Can you work these out from the drawing? Everything is in mm from the part's minimum corner. A direction names the side the tool comes from. Round coordinates to 2 decimals unless told otherwise and drop trailing zeros. Loops run counter-clockwise (first coordinate to the right, second up) from the corner with the lowest first, then second, coordinate; pieces in that order, holes last. Notation, with made-up numbers: (14.5, -2) -> (58.5, -2) arc R15 cw to (58.5, 9) -> close; hole circle Ø4 at (39.25, 29). An arc over 180 degrees is marked (long way). One line per item, written item: value.
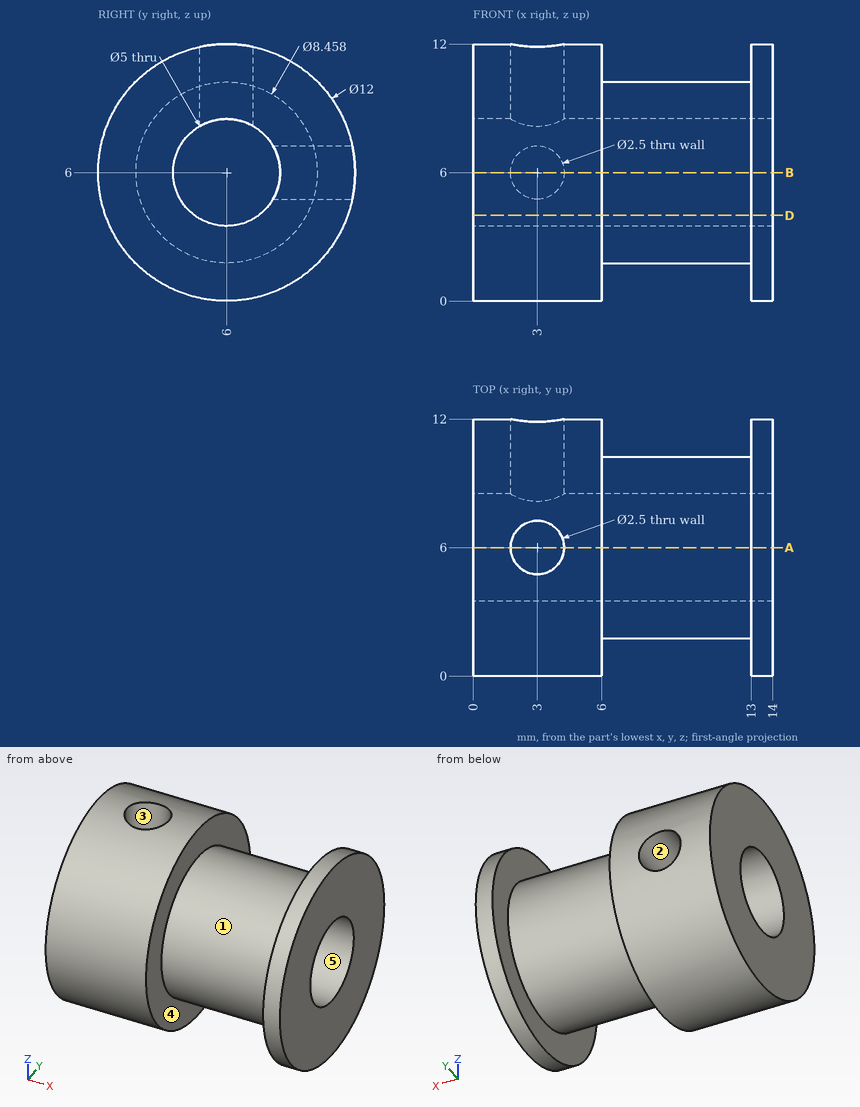
Item 1: If we section it at A-A on y = 6: List the corners of the cut face in (x, z) for me.
Output:
outline: (0, 0) -> (6, 0) -> (6, 1.77) -> (13, 1.77) -> (13, 0) -> (14, 0) -> (14, 3.5) -> (0, 3.5) -> close; (0, 8.5) -> (1.75, 8.5) -> (1.75, 12) -> (0, 12) -> close; (4.25, 8.5) -> (14, 8.5) -> (14, 12) -> (13, 12) -> (13, 10.23) -> (6, 10.23) -> (6, 12) -> (4.25, 12) -> close
Item 2: For the marked faces 4 and 5, which set-ups out of +Z, -Z, +X, -X, +Y, -Y let a thin tool reach every point of the face, with its end or its side?
Output:
face 4: none
face 5: +X, -X
Item 3: I need wall thicknesses on line 1 (X direction, y = 6, z = 9.9); line 2 (X direction, y = 4, z = 0.5); line 3 (Y direction, x = 2, z = 8.75). Which ranges of each line are inside material? Lowest first, please. Write a range as from..to.
Output:
line 1: x = 0..1.75, 4.25..14
line 2: x = 0..6, 13..14
line 3: y = 0.67..5.25, 6.75..11.33
Item 4: If we section it at D-D on z = 4: List the corners of the cut face in (x, y) for me.
Output:
outline: (0, 0.34) -> (6, 0.34) -> (6, 2.27) -> (13, 2.27) -> (13, 0.34) -> (14, 0.34) -> (14, 4.5) -> (0, 4.5) -> close; (0, 7.5) -> (14, 7.5) -> (14, 11.66) -> (13, 11.66) -> (13, 9.73) -> (6, 9.73) -> (6, 11.66) -> (0, 11.66) -> close
Item 5: If we mould it in two halves opening along Z, with no side actions, what happens to the marked faces 1, 2 and 3? For each: released by +Z, released by -Z, zero draft, split by the parting line, or undercut.
Output:
face 1: split by the parting line
face 2: undercut
face 3: zero draft
Item 6: Will these pins go through, and if not, where does the flat tip stop? pin 1 Ø1.5 at (x, y) = (9, 1.5) entering from -Z (1 decimal); pin 2 Ø6 at (x, y) = (9.5, 9) entering from -Z; pin 3 Ø2 at (x, z) = (10.5, 5) entering from +Y.
Output:
pin 1: stops at z = 4
pin 2: stops at z = 1.77
pin 3: stops at y = 10.23
